```python
from build123d import *

# Parameters (mm, degrees)
SKETCH1_R           = 1.75
BOSS_EXTRUDE1_DEPTH = 0.75
FILLET1_R           = 2
FILLET2_R           = 0.5
SKETCH2_W           = 0.6
SKETCH2_H           = 1.5
BOSS_EXTRUDE2_DEPTH = 0.15
FILLET3_R           = 0.05


with BuildPart() as part:
    # Sketch1 → Boss-Extrude1 (new, symmetric)
    with BuildSketch(Plane(origin=(0, 0, 0), x_dir=(1, 0, 0), z_dir=(0, 1, 0))):
        with BuildLine():
            Line((-2.5, 12), (-2.5, 0))
            Line((-2.5, 0), (-4.689391033, -1.145712258))
            Line((-4.689391033, -1.145712258), (4.608210726, -21.084483573))
            ThreePointArc((4.608210726, -21.084483573), (9.259451896, -22.777396911), (10.952365235, -18.126155741))
            Line((10.952365235, -18.126155741), (2.5, 0))
            Line((2.5, 0), (2.5, 15))
            Line((2.5, 15), (-1.891164992, 19.391164992))
            Line((-1.891164992, 19.391164992), (-6.891164992, 19.391164992))
            Line((-6.891164992, 19.391164992), (-6.891164992, 14.391164992))
            Line((-6.891164992, 14.391164992), (-2.5, 12))
        make_face()
        with Locations(Location((-3.891164992, 16.391164992, 0), (0, 0, 270))):
            Circle(SKETCH1_R, mode=Mode.SUBTRACT)
        with Locations(Location((0, -2.5, 0), (0, 0, 270))):
            Circle(SKETCH1_R, mode=Mode.SUBTRACT)
        with Locations(Location((7.78028798, -19.605319657, 0), (0, 0, 270))):
            Circle(SKETCH1_R, mode=Mode.SUBTRACT)
    extrude(amount=BOSS_EXTRUDE1_DEPTH, both=True)

    # Fillet1
    fillet1_edges = [part.edges().sort_by_distance(p)[0] for p in [
        (2.5, 0, -15),
        (-4.689391033, 0, 1.145712258),
    ]]
    fillet(fillet1_edges, radius=FILLET1_R)

    # Fillet2
    fillet2_edges = [part.edges().sort_by_distance(p)[0] for p in [
        (-1.891164992, 0, -19.391164992),
        (2.5, 0, 0),
        (-2.5, 0, -12),
    ]]
    fillet(fillet2_edges, radius=FILLET2_R)

    # Sketch2 → Boss-Extrude2 (add)
    with BuildSketch(Plane.ZY.offset(6.891164992)):
        with Locations((-14.691164992, 0)):
            Rectangle(SKETCH2_W, SKETCH2_H)
        with Locations((-15.691164992, 0)):
            Rectangle(SKETCH2_W, SKETCH2_H)
        with Locations((-16.691164992, 0)):
            Rectangle(SKETCH2_W, SKETCH2_H)
        with Locations((-17.691164992, 0)):
            Rectangle(SKETCH2_W, SKETCH2_H)
        with Locations((-18.691164992, 0)):
            Rectangle(SKETCH2_W, SKETCH2_H)
    extrude(amount=BOSS_EXTRUDE2_DEPTH)

    # Fillet3
    fillet3_edges = [part.edges().sort_by_distance(p)[0] for p in [
        (-7.041164992, 0, -16.991164992),
        (-7.041164992, 0, -16.391164992),
        (-7.041164992, 0, -17.991164992),
        (-7.041164992, 0, -17.391164992),
        (-7.041164992, 0, -18.991164992),
        (-7.041164992, 0, -18.391164992),
        (-7.041164992, 0, -14.991164992),
        (-7.041164992, 0, -14.391164992),
        (-7.041164992, 0, -15.991164992),
        (-7.041164992, 0, -15.391164992),
    ]]
    fillet(fillet3_edges, radius=FILLET3_R)


solid = part.part
```
Geometry check sheet. Reference: the model listing, model coordinates, mm. A direction names the side the tool comes from. Coordinates: 2 decimals unless noted, no trailing zeros. Loops run counter-clockwise (first coordinate to the right, second up) from the corner with the lowest first, then second, coordinate; pieces in that order, holes last.
Item 1: Thickness scan on line 1 (Z direction, x = -3, y = 0); line 2 (Z direction, x = -1, y = -0.3); line 3 (X direction, y = -0.35, z = -6). Record the ranges inside material, lowest first.
Item 2: Release check for a two-part mould opening along Z. For faces 1 (the face through (-4, 0, -19.391)), 2 (the face through (-2.5, 0, -6)), 3 (the face through (0.3, 0.01, 11.85)), 4 (the face through (2, 0.75, 2)) record: released by +Z, released by -Z, zero draft, split by the parting line, or undercut.
Item 3: Sectioned sample at C-C, the plane y = -0.1. Count the separate pieces of the cut face and the enclosed holes in it, then the cut area to 3 significant figures.
Item 4: Access from +Z, -Z, +X, -X, +Y, -Y to the whole of each face (thin tool, end or side, straight path). Record for faces 5 (the face through (2.5, 0, -7)), 6 (the face through (-0.67, -0.01, 4.117)), 7 (the face through (-4.85, 0.01, -13.28)).
Item 5: Go/stop test with a flat-tipped pin: pin 1 Ø3 at (x, z) = (3.5, -0.5) entering from +Y. Record where the tip stops, or that it passes through.
Item 6: Sectioned sample at B-B, the plane x = 0. Record the boundary of the cut face in (y, z).
Item 7: Sectioned sample at A-A, the plane z = 2.5. Record the boundary of the cut face in (x, y).
Check result:
1. line 1: z = -19.39 to -17.9, -14.89 to -12.27, 0.26 to 4.77
1. line 2: z = -18.5 to 1.06, 3.94 to 9.06
1. line 3: x = -2.5 to 2.5
2. face 1: released by -Z
2. face 2: undercut
2. face 3: released by +Z
2. face 4: zero draft
3. separate pieces: 1
3. enclosed holes: 3
3. area: 254 mm2
4. face 5: -Z, +X, +Y, -Y
4. face 6: +Y, -Y
4. face 7: -X, +Y, -Y
5. pin 1: stops at y = 0.75
6. outline: (-0.75, -17.5) - (0.75, -17.5) - (0.75, 0.75) - (-0.75, 0.75) - close; (-0.75, 4.25) - (0.75, 4.25) - (0.75, 11.2) - (-0.75, 11.2) - close
7. outline: (-4.01, -0.75) - (-1.75, -0.75) - (-1.75, 0.75) - (-4.01, 0.75) - close; (1.75, -0.75) - (3.67, -0.75) - (3.67, 0.75) - (1.75, 0.75) - close
